```python
from build123d import *

# Parameters (mm, degrees)
BOSS_EXTRUDE1_DEPTH  = 25
BOSS_EXTRUDE2_DEPTH  = 2.5
SKETCH5_W            = 20
SKETCH5_H            = 7.5
SKETCH5_W_2          = 7.54
SKETCH5_H_2          = 3.54
SKETCH5_W_3          = 3.54
BOSS_EXTRUDE3_DEPTH  = 10
SKETCH6_R            = 1.0485
CUT_EXTRUDE1_DEPTH   = 39.259802665
FILLET1_R            = 2
M2_CLEARANCE_HOLE1_D = 2.6
SKETCH9_R            = 2.05
CUT_EXTRUDE4_DEPTH   = 38.186186952
SKETCH10_W           = 12.5
SKETCH10_H           = 55
CUT_EXTRUDE5_DEPTH   = 2.5
CHAMFER1_SIZE        = 2.5


with BuildPart() as part:
    # Sketch2 → Boss-Extrude1 (new, symmetric)
    with BuildSketch(Plane.XY):
        Polygon((10, -2.5), (10, -18.75), (16, -18.75), (10, 2.5), (-10, 2.5), (-16, -18.75), (-10, -18.75), (-10, -2.5), align=None)
    extrude(amount=BOSS_EXTRUDE1_DEPTH, both=True)

    # Sketch3 → Boss-Extrude2 (add)
    with BuildSketch(Plane.XY.offset(25)):
        Polygon((-10, -18.75), (10, -18.75), (16, -18.75), (10, 2.5), (-10, 2.5), (-16, -18.75), align=None)
    boss_extrude2 = extrude(amount=BOSS_EXTRUDE2_DEPTH)

    # Mirror1: Boss-Extrude2 across plane
    add(boss_extrude2.mirror(Plane.XY))

    # Sketch5 → Boss-Extrude3 (add)
    # profile 1 of 2: a face of its own
    with BuildSketch(Plane.XZ.offset(2.5)):
        with Locations((0, 21.25)):
            Rectangle(SKETCH5_W, SKETCH5_H)
        with Locations((0, 21.75)):
            Rectangle(SKETCH5_W_2, SKETCH5_H_2, mode=Mode.SUBTRACT)
    # profile 2 of 2: a face of its own
    with BuildSketch(Plane.XZ.offset(2.5)):
        with Locations((0, -21.25)):
            Rectangle(SKETCH5_W, SKETCH5_H)
        with Locations((-2, -21.75)):
            Rectangle(SKETCH5_W_3, SKETCH5_H_2, mode=Mode.SUBTRACT)
    extrude(amount=BOSS_EXTRUDE3_DEPTH)

    # Sketch6 → Cut-Extrude1 (cut, through all)
    with BuildSketch(Plane(origin=(0, 2.5, 0), x_dir=(1, 0, 0), z_dir=(0, 1, 0))):
        with Locations(Location((-2, 21.75, 0), (0, 0, 270))):
            Circle(SKETCH6_R)
        with Locations(Location((-2, -21.75, 0), (0, 0, 270))):
            Circle(SKETCH6_R)
        with Locations(Location((2, -21.75, 0), (0, 0, 270))):
            Circle(SKETCH6_R)
    extrude(amount=-CUT_EXTRUDE1_DEPTH, mode=Mode.SUBTRACT)

    # Fillet1
    fillet1_edges = [part.edges().sort_by_distance(p)[0] for p in [
        (-10, 2.5, 0),
        (10, 2.5, 0),
        (10, -2.5, 0),
        (-10, -2.5, 0),
        (0, -12.5, 17.5),
        (0, -12.5, -17.5),
    ]]
    fillet(fillet1_edges, radius=FILLET1_R)

    # M2 Clearance Hole1 (through all)
    with Locations(Plane.XZ.offset(18.75)):
        with Locations((-13, 17.5), (13, 17.5), (13, -17.5), (-13, -17.5)):
            Hole(M2_CLEARANCE_HOLE1_D / 2)

    # Sketch9 → Cut-Extrude4 (cut, through all)
    with BuildSketch(Plane.XZ.offset(16.75)):
        with Locations((-13, -17.5)):
            Circle(SKETCH9_R)
        with Locations((13, -17.5)):
            Circle(SKETCH9_R)
        with Locations((13, 17.5)):
            Circle(SKETCH9_R)
        with Locations((-13, 17.5)):
            Circle(SKETCH9_R)
    extrude(amount=-CUT_EXTRUDE4_DEPTH, mode=Mode.SUBTRACT)

    # Sketch10 → Cut-Extrude5 (cut)
    with BuildSketch(Plane(origin=(0, 2.5, 0), x_dir=(1, 0, 0), z_dir=(0, 1, 0))):
        Rectangle(SKETCH10_W, SKETCH10_H)
    extrude(amount=-CUT_EXTRUDE5_DEPTH, mode=Mode.SUBTRACT)

    # Chamfer1
    # the kernel refuses this chamfer: 2.5 mm, written as the material it takes off along each edge
    with BuildSketch(Plane(origin=(6.25, 2.5, 33.92920747), x_dir=(-0.027495876610586317, -0.9996219169112968, 0), z_dir=(0, 0, -1))) as chamfer1_piece_1_section:
        Polygon((CHAMFER1_SIZE * 0.999621916911, -CHAMFER1_SIZE * 0.0274958766106), (-CHAMFER1_SIZE * 0.0274958766106, -CHAMFER1_SIZE * 0.999621916911), (0, 0), align=None)
    chamfer1_piece_1 = extrude(amount=67.85841494, mode=Mode.PRIVATE)
    chamfer1_piece_1 = split(chamfer1_piece_1, bisect_by=Plane(origin=(7.076010386, 0, 0), z_dir=(0, 1, 0)), keep=Keep.TOP, mode=Mode.PRIVATE)
    add(chamfer1_piece_1, mode=Mode.SUBTRACT)
    with BuildSketch(Plane(origin=(-6.25, 2.5, -33.92920747), x_dir=(-0.9996219169112968, 0.02749587661058649, 0), z_dir=(0, 0, 1))) as chamfer1_piece_2_section:
        Polygon((CHAMFER1_SIZE * 0.999621916911, CHAMFER1_SIZE * 0.0274958766106), (-CHAMFER1_SIZE * 0.0274958766106, CHAMFER1_SIZE * 0.999621916911), (0, 0), align=None)
    chamfer1_piece_2 = extrude(amount=67.85841494, mode=Mode.PRIVATE)
    chamfer1_piece_2 = split(chamfer1_piece_2, bisect_by=Plane(origin=(-7.076010386, 0, 0), z_dir=(0, 1, 0)), keep=Keep.TOP, mode=Mode.PRIVATE)
    add(chamfer1_piece_2, mode=Mode.SUBTRACT)


solid = part.part
```
The model under review builds one solid part; all positions refer to its coordinate system, in mm. A direction names the side the tool comes from. Round coordinates to 2 decimals unless told otherwise and drop trailing zeros. Order: outer loops, then holes, each group sorted by start corner. A loop starts at its lowest first (then second) coordinate and runs counter-clockwise, first axis right, second up. Notation, with made-up numbers: (4.5, 82.25) -> (20.5, 82.25) arc R14 ccw to (20.5, 93.25) -> close; hole circle Ø1 at (24, -33.75). An arc over 180 degrees is marked (long way). One line per item, written item: value. Start each with the question number.
Q1. Take a section at B-B (z = -21.75). Write out the cut boundary in (x, y).
Q2. Mouldability with a two-part tool opening along Z and no side actions: class faces 1 (the face through (-2, -1.2, 20.7)), 2 (the face through (7.47, 1.22, 0.38)) as released by +Z, released by -Z, zero draft, split by the parting line, or undercut.
Q3. Machinability: for faces 3 (the face through (-7.51, 1.26, -0.38)), 4 (the face through (11.76, -17.74, -17.11)), 5 (the face through (0, -7, 23.52)), 6 (the face through (13, -16.75, -19)), which of the approach directions +Z, -Z, +X, -X, +Y, -Y give a long, thin tool a straight path to every point of the face, cutting with its end or side? Answer none if there is none.
Q4. Take a section at C-C (x = 13). Write out the cut boundary in (y, z) (3 decimals).
Q5. Wall thickness on line 1 (Z direction, x = 13, y = -18.2); line 2 (Z direction, x = 13, y = -11.25); line 3 (X direction, y = -16, z = -16.5): over which ranges is each line inside the solid? List them lowest first.
Q6. Take a section at A-A (x = 2). Write out the cut boundary in (y, z), and give its area (3 significant figures).
Q7. Clearance check with flat-ended pins moving along their axes: pin 1 Ø4 at (x, z) = (7.5, 18.5) entering from -Y; pin 2 Ø8 at (x, z) = (-2, -1.5) entering from +Y; pin 3 Ø3.5 at (x, z) = (13, -17.5) entering from +Y. State where each tip first meets the part, or that it passes through.
Q8. Take a section at D-D (y = -13.75). Write out the cut boundary in (x, z).
Reported:
1. outline: (-16, -18.75) -> (-10, -18.75) -> (-10, -12.5) -> (-3.77, -12.5) -> (-3.77, -2.5) -> (-3.05, -2.5) -> (-3.05, 0) -> (-6.25, 0) -> (-8.73, 2.48) arc R2 ccw to (-10.41, 1.04) -> close; (-0.95, -2.5) -> (-0.23, -2.5) -> (-0.23, -12.5) -> (10, -12.5) -> (10, -18.75) -> (16, -18.75) -> (10.41, 1.04) arc R2 ccw to (8.73, 2.48) -> (6.25, 0) -> (-0.95, 0) -> close
2. face 1: undercut
2. face 2: zero draft
3. face 3: +Z, -Z, +Y
3. face 4: +Y, -Y
3. face 5: -Y
3. face 6: +Y
4. outline: (-18.75, -27.5) -> (-8.125, -27.5) -> (-8.125, -19.55) -> (-16.75, -19.55) -> (-16.75, -18.8) -> (-18.75, -18.8) -> close; (-18.75, -16.2) -> (-16.75, -16.2) -> (-16.75, -15.45) -> (-8.125, -15.45) -> (-8.125, 15.45) -> (-16.75, 15.45) -> (-16.75, 16.2) -> (-18.75, 16.2) -> close; (-18.75, 18.8) -> (-16.75, 18.8) -> (-16.75, 19.55) -> (-8.125, 19.55) -> (-8.125, 27.5) -> (-18.75, 27.5) -> close
5. line 1: z = -27.5 to -18.8, -16.2 to 16.2, 18.8 to 27.5
5. line 2: z = -27.5 to -19.55, -15.45 to 15.45, 19.55 to 27.5
5. line 3: x = -15.22 to -14.79, -11.21 to -10, 10 to 11.21, 14.79 to 15.22
6. outline: (-18.75, -27.5) -> (0, -27.5) -> (0, 20.7) -> (-2.5, 20.7) -> (-2.5, 19.98) -> (-12.5, 19.98) -> (-12.5, 19.5) arc R2 ccw to (-10.5, 17.5) -> (-2.5, 17.5) -> (-2.5, -17.5) -> (-10.5, -17.5) arc R2 ccw to (-12.5, -19.5) -> (-12.5, -25) -> (-18.75, -25) -> close; (-18.75, 25) -> (-12.5, 25) -> (-12.5, 23.52) -> (-2.5, 23.52) -> (-2.5, 22.8) -> (0, 22.8) -> (0, 27.5) -> (-18.75, 27.5) -> close
6. area: 326 mm2
7. pin 1: stops at y = -12.5
7. pin 2: stops at y = 0
7. pin 3: stops at y = -16.75
8. outline: (-14.59, -27.5) -> (14.59, -27.5) -> (14.59, -18.8) arc R2.05 cw (long way) to (14.59, -16.2) -> (14.59, 16.2) arc R2.05 cw (long way) to (14.59, 18.8) -> (14.59, 27.5) -> (-14.59, 27.5) -> (-14.59, 18.8) arc R2.05 cw (long way) to (-14.59, 16.2) -> (-14.59, -16.2) arc R2.05 cw (long way) to (-14.59, -18.8) -> close; hole (-10, -25) -> (10, -25) -> (10, 25) -> (-10, 25) -> close
